```python
from build123d import *

# Parameters (mm, degrees)
F3_D           = 12.25
F3_CSINK_D     = 13.5
F3_CSINK_ANGLE = 60


with BuildPart() as f1:
    # F0 (on Front) → F1 (revolve)
    with BuildSketch(Plane.XZ):
        with BuildLine():
            Line((10.1, 0), (0, 0))
            Line((0, 0), (0, -15.5))
            Line((0, -15.5), (8, -15.5))
            Line((8, -15.5), (9.81555, -2.099511))
            ThreePointArc((9.81555, -2.099511), (9.829834, -1.961906), (9.85268, -1.82546))
            Line((9.85268, -1.82546), (10.1, 0))
        make_face()
        with BuildLine():
            Line((11.908681, -0.047055), (10.1, 0))
            Line((10.1, 0), (9.85268, -1.82546))
            ThreePointArc((9.85268, -1.82546), (10.575835, -0.583828), (11.908681, -0.047055))
        make_face()
    revolve(axis=Axis((0, 0, -7.75), (0, 0, -1)))

    # F3 (through all)
    with Locations(Plane.XY):
        with Locations((0, -1.75)):
            CounterSinkHole(F3_D / 2, F3_CSINK_D / 2, counter_sink_angle=F3_CSINK_ANGLE)


solid = f1.part
```
Check sheet for the modelled part. Datum: model origin and axes. Units: mm. Give positions to 0.01 mm unless a question says otherwise; leave off trailing zeros. Write each loop counter-clockwise with the first axis right and the second up, starting at its lowest first coordinate (ties: lowest second). Pieces come first, ordered by that corner, then holes. Notation, with made-up numbers: (-21, -1) - (28, -1) arc R18 cw to (28, 32) - close; hole circle Ø4 at (60.5, -10.75). An arc over 180 degrees is marked (long way). Answer as a JSON object with one key per item and string values. Group by question number.
1) Sectioned sample at B-B (z = -5). Record the cut outline in (x, y) (3 decimals).
2) Sectioned sample at C-C (z = -14). Record the cut outline in (x, y) (3 decimals).
3) Depth check by flat-ended pin: P1, Ø1, axis at x = -9, z = -4.5, coming from the -Y side; P2, Ø1, axis at y = -8.5, z = -5, coming from the +X side; P3, Ø2, axis at y = 9, z = -6.5, coming from the +X side. Enter the tip coordinate at first touch or a pass-through.
4) Thickness scan on probe 1 along X at (y, z) = (-1.75, -5) (3 decimals); probe 2 along Y at (x, z) = (0, -9.5) (3 decimals); probe 3 along Y at (x, z) = (0, -12.25) (3 decimals). Record the ranges inside material, lowest first. Write a range as from..to.
5) Sectioned sample at A-A (x = 0). Record the cut outline in (y, z) (3 decimals), then the cut area to 3 significant figures.
6) Release check for a two-part mould opening along X. For faces 1 (the face through (8.316, -2.619, -10.195)), 2 (the face through (1, 5, -15.5)), 3 (the face through (-5.84, 0.09, -8.39)) record: pulls with the +X half, pulls with the -X half, needs draft (parallel to the pull), parting line crosses it, or undercut.
Geometry results:
{
 "1": {"outline": "circle Ø18.845 at (0, 0); hole circle Ø12.25 at (0, -1.75)"},
 "2": {"outline": "circle Ø16.406 at (0, 0); hole circle Ø12.25 at (0, -1.75)"},
 "3": {"P1": "stops at y = -4.23", "P2": "stops at x = 4.99", "P3": "stops at x = 4.6"},
 "4": {"probe 1": "x = -9.259..-6.125, 6.125..9.259", "probe 2": "y = -8.813..-7.875, 4.375..8.813", "probe 3": "y = -8.44..-7.875, 4.375..8.44"},
 "5": {"outline": "(-11.909, -0.047) arc R2.215 cw to (-9.853, -1.825) arc R2.215 cw to (-9.816, -2.1) - (-8, -15.5) - (-7.875, -15.5) - (-7.875, -1.083) - (-8.5, 0) - (-10.1, 0) - close; (4.375, -15.5) - (8, -15.5) - (9.816, -2.1) arc R2.215 cw to (9.853, -1.825) arc R2.215 cw to (11.909, -0.047) - (10.1, 0) - (5, 0) - (4.375, -1.083) - close", "area": "91.6 mm^2"},
 "6": {"face 1": "parting line crosses it", "face 2": "needs draft", "face 3": "undercut"}
}
